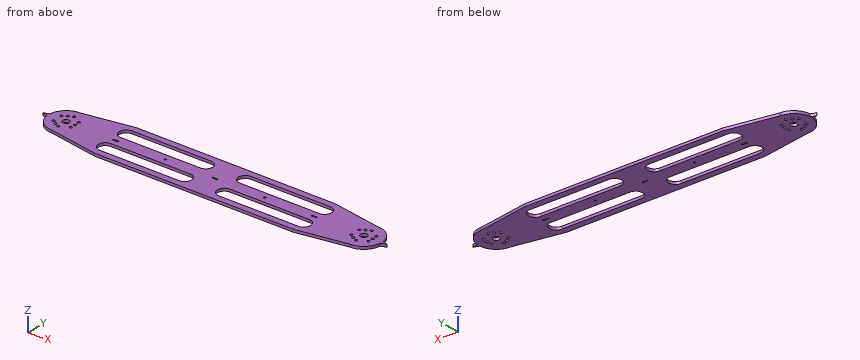
from build123d import *

# Parameters (mm, degrees)
SKETCH_1_R      = 2
SKETCH_1_R_2    = 2.05
SKETCH_1_R_3    = 5
SKETCH_1_R_4    = 1.5
SKETCH_1_W      = 8.2
SKETCH_1_H      = 2.2
EXTRUDE_1_DEPTH = 4


with BuildPart() as part:
    # 草图1 → 凸台-拉伸1 (new body)
    with BuildSketch(Plane.XY):
        with BuildLine():
            Line((375, 40), (450, 27))
            Line((450, 27), (452.35435733, 26.897156013))
            ThreePointArc((452.35435733, 26.897156013), (468.941976287, 19.240621984), (476.857038268, 2.774796472))
            Line((476.857038268, 2.774796472), (485, 0))
            Line((485, 0), (476.857038268, -2.774796472))
            ThreePointArc((476.857038268, -2.774796472), (468.941976287, -19.240621984), (452.35435733, -26.897156013))
            Line((452.35435733, -26.897156013), (450, -27))
            Line((450, -27), (375, -40))
            Line((375, -40), (75, -40))
            Line((75, -40), (0, -27))
            Line((0, -27), (-2.35435733, -26.897156013))
            ThreePointArc((-2.35435733, -26.897156013), (-18.941976287, -19.240621984), (-26.857038268, -2.774796472))
            Line((-26.857038268, -2.774796472), (-35, 0))
            Line((-35, 0), (-26.857038268, 2.774796472))
            ThreePointArc((-26.857038268, 2.774796472), (-18.941976287, 19.240621984), (-2.35435733, 26.897156013))
            Line((-2.35435733, 26.897156013), (0, 27))
            Line((0, 27), (75, 40))
            Line((75, 40), (375, 40))
        make_face()
        with Locations((0, -15)):
            Circle(SKETCH_1_R, mode=Mode.SUBTRACT)
        with Locations((-12.990381057, -7.5)):
            Circle(SKETCH_1_R, mode=Mode.SUBTRACT)
        with Locations((-12.990381057, 7.5)):
            Circle(SKETCH_1_R, mode=Mode.SUBTRACT)
        with Locations((0, 15)):
            Circle(SKETCH_1_R, mode=Mode.SUBTRACT)
        with Locations((12.990381057, 7.5)):
            Circle(SKETCH_1_R, mode=Mode.SUBTRACT)
        with Locations((12.990381057, -7.5)):
            Circle(SKETCH_1_R, mode=Mode.SUBTRACT)
        with Locations((13.53, 0)):
            Circle(SKETCH_1_R_2, mode=Mode.SUBTRACT)
        with Locations((-6.765, -11.717323713)):
            Circle(SKETCH_1_R_2, mode=Mode.SUBTRACT)
        with Locations((-6.765, 11.717323713)):
            Circle(SKETCH_1_R_2, mode=Mode.SUBTRACT)
        Circle(SKETCH_1_R_3, mode=Mode.SUBTRACT)
        with Locations((450, -15)):
            Circle(SKETCH_1_R, mode=Mode.SUBTRACT)
        with Locations((437.009618943, -7.5)):
            Circle(SKETCH_1_R, mode=Mode.SUBTRACT)
        with Locations((437.009618943, 7.5)):
            Circle(SKETCH_1_R, mode=Mode.SUBTRACT)
        with Locations((450, 15)):
            Circle(SKETCH_1_R, mode=Mode.SUBTRACT)
        with Locations((462.990381057, 7.5)):
            Circle(SKETCH_1_R, mode=Mode.SUBTRACT)
        with Locations((462.990381057, -7.5)):
            Circle(SKETCH_1_R, mode=Mode.SUBTRACT)
        with Locations((463.53, 0)):
            Circle(SKETCH_1_R_2, mode=Mode.SUBTRACT)
        with Locations((443.235, -11.717323713)):
            Circle(SKETCH_1_R_2, mode=Mode.SUBTRACT)
        with Locations((443.235, 11.717323713)):
            Circle(SKETCH_1_R_2, mode=Mode.SUBTRACT)
        with Locations((450, 0)):
            Circle(SKETCH_1_R_3, mode=Mode.SUBTRACT)
        with Locations((300, 0)):
            Circle(SKETCH_1_R_4, mode=Mode.SUBTRACT)
        with Locations((150, 0)):
            Circle(SKETCH_1_R_4, mode=Mode.SUBTRACT)
        with Locations((225, 0)):
            Rectangle(SKETCH_1_W, SKETCH_1_H, mode=Mode.SUBTRACT)
        with Locations((75, 0)):
            Rectangle(SKETCH_1_W, SKETCH_1_H, mode=Mode.SUBTRACT)
        with Locations((375, 0)):
            Rectangle(SKETCH_1_W, SKETCH_1_H, mode=Mode.SUBTRACT)
        with BuildLine():
            Line((75, 30.5), (195, 30.5))
            ThreePointArc((195, 30.5), (205.5, 20), (195, 9.5))
            Line((195, 9.5), (75, 9.5))
            ThreePointArc((75, 9.5), (64.5, 20), (75, 30.5))
        make_face(mode=Mode.SUBTRACT)
        with BuildLine():
            Line((375, 30.5), (255, 30.5))
            ThreePointArc((255, 30.5), (244.5, 20), (255, 9.5))
            Line((255, 9.5), (375, 9.5))
            ThreePointArc((375, 9.5), (385.5, 20), (375, 30.5))
        make_face(mode=Mode.SUBTRACT)
        with BuildLine():
            Line((75, -30.5), (195, -30.5))
            ThreePointArc((195, -30.5), (205.5, -20), (195, -9.5))
            Line((195, -9.5), (75, -9.5))
            ThreePointArc((75, -9.5), (64.5, -20), (75, -30.5))
        make_face(mode=Mode.SUBTRACT)
        with BuildLine():
            Line((375, -30.5), (255, -30.5))
            ThreePointArc((255, -30.5), (244.5, -20), (255, -9.5))
            Line((255, -9.5), (375, -9.5))
            ThreePointArc((375, -9.5), (385.5, -20), (375, -30.5))
        make_face(mode=Mode.SUBTRACT)
    extrude(amount=EXTRUDE_1_DEPTH)


solid = part.part
Could you check a few things on this model? Use its own coordinates, in mm. Give positions to 0.01 mm unless a question says otherwise; leave off trailing zeros. Order: outer loops, then holes, each group sorted by start corner. A loop starts at its lowest first (then second) coordinate and runs counter-clockwise, first axis right, second up. Notation, with made-up numbers: (27, -1.75) - (68, -1.75) arc R6 cw to (68, 3.25) - close; hole circle Ø5 at (9, -13.5). An arc over 180 degrees is marked (long way). Return JSON: item names as keys, results as strings. Group by question number.
Q1. Please list where these lines run through material, in increasing order: line 1 along Y through (x, z) = (278.5, 0.3); line 2 along Y through (x, z) = (450, 1.95); line 3 along X through (y, z) = (4, 2). Write a range as [from, to].
Q2. Suppose I cut it at B-B, the plane z = 1.3. State how many separate pieces and enclosed holes the cut face has, and give its area (3 significant figures).
Q3. Will these pins go through, and if not, where does the flat tip stop? pin 1 Ø1.5 at (x, z) = (395, 1.5) entering from -Y; pin 2 Ø1.8 at (y, z) = (0, 1.5) entering from +X; pin 3 Ø1.5 at (x, z) = (423, 1.5) entering from -Y; pin 4 Ø3 at (x, y) = (-12.99, -7.5) entering from +Z.
Q4. Suppose I cut it at A-A, the plane x = 320. Please give me the cut outline in (y, z).
Resolved:
{
 "1": {"line 1": "y = [-40, -30.5], [-9.5, 9.5], [30.5, 40]", "line 2": "y = [-27, -17], [-13, -5], [5, 13], [17, 27]", "line 3": "x = [-26.7, -3], [3, 447], [453, 476.7]"},
 "2": {"separate pieces": "1", "enclosed holes": "29", "area": "24,500 mm2"},
 "3": {"pin 1": "stops at y = -36.66", "pin 2": "stops at x = 485", "pin 3": "stops at y = -31.81", "pin 4": "passes through"},
 "4": {"outline": "(-40, 0) - (-30.5, 0) - (-30.5, 4) - (-40, 4) - close; (-9.5, 0) - (9.5, 0) - (9.5, 4) - (-9.5, 4) - close; (30.5, 0) - (40, 0) - (40, 4) - (30.5, 4) - close"}
}
